Check sheet for the modelled part. Datum: model origin and axes. Units: mm. Face numbers are marked on the shaded views. A direction names the side the tool comes from. Round coordinates to 2 decimals unless told otherwise and drop trailing zeros. Order: outer loops, then holes, each group sorted by start corner. A loop starts at its lowest first (then second) coordinate and runs counter-clockwise, first axis right, second up. Notation, with made-up numbers: M 26,17 L 48,17 A28 ccw 48,47 Z; hole C 7,65.25 d2. An arc over 180 degrees is marked long. One line per item, written item: value. Start each with the question number.
(1) Cross-section at B-B, the plane y = -8. Enter the section's corners in (x, z), and give its area (3 significant figures).
(2) Depth check by flat-ended pin: pin 1 Ø1.5 at (x, y) = (8, -26) entering from +Z; pin 2 Ø1.5 at (x, z) = (3.5, 2) entering from +Y; pin 3 Ø0.9 at (y, z) = (1.5, 1.5) entering from +X; pin 4 Ø0.9 at (x, z) = (1.5, 1.5) entering from -Y. Enter the tip coordinate at first touch or a pass-through.
(3) Release check for a two-part mould opening along X. For the marked faces 1, 2 and 3 record: released by +X, released by -X, zero draft, split by the parting line, or undercut.
(4) Cross-section at A-A, the plane x = 10.2. Enter the section's corners in (y, z), and give its area (3 significant figures).
(5) Cross-section at C-C, the plane z = 2.2. Enter the section's corners in (x, y).
(6) Cross-section at D-D, the plane y = -26. Enter the section's corners in (x, z), and give its area (3 significant figures).
(7) Thickness scan on L1, parallel to Y at x = 10.2, z = 1.95; L2, parallel to X at y = -7.5, z = 1.5; L3, parallel to X at y = 1.5, z = 2.7. Record the ranges inside material, lowest first.
(8) Access from +Z, -Z, +X, -X, +Y, -Y to the whole of each face (thin tool, end or side, straight path). Record for the marked faces 4, 5, 6, 7 and 8.
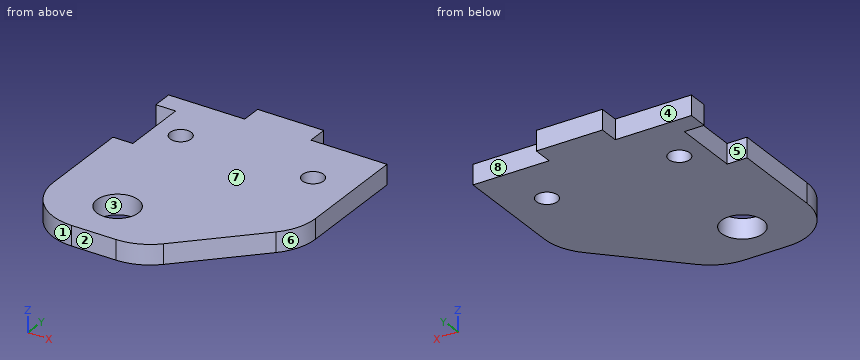
from build123d import *

# Parameters (mm, degrees)
ESBO_O1_R                = 1.6
ESBO_O1_R_2              = 3.15
RESSALTO_EXTRUS_O1_DEPTH = 3
CHANFRO2_SIZE            = 15
FILETE2_R                = 8


with BuildPart() as part:
    # Esboço1 → Ressalto-extrusão1 (new body)
    with BuildSketch(Plane.XY):
        Polygon((11.5, 0), (0, 0), (0, -3), (3, -3), (3, -13), (0, -13), (0, -35), (33, -35), (33, 0), (21.5, 0), (21.5, 3), (11.5, 3), align=None)
        with Locations((27, -8)):
            Circle(ESBO_O1_R, mode=Mode.SUBTRACT)
        with Locations((7, -8)):
            Circle(ESBO_O1_R, mode=Mode.SUBTRACT)
        with Locations((10.2, -27.684295139)):
            Circle(ESBO_O1_R_2, mode=Mode.SUBTRACT)
    extrude(amount=RESSALTO_EXTRUS_O1_DEPTH)

    # Chanfro2
    chanfro2_edges = [part.edges().sort_by_distance(p)[0] for p in [
        (33, -35, 1.5),
    ]]
    chamfer(chanfro2_edges, length=CHANFRO2_SIZE)

    # Filete2
    filete2_edges = [part.edges().sort_by_distance(p)[0] for p in [
        (0, -35, 1.5),
        (33, -20, 1.5),
        (18, -35, 1.5),
    ]]
    fillet(filete2_edges, radius=FILETE2_R)


solid = part.part
Values found:
1. outline: M 3,0 L 5.4,0 L 5.4,3 L 3,3 Z; M 8.6,0 L 25.4,0 L 25.4,3 L 8.6,3 Z; M 28.6,0 L 33,0 L 33,3 L 28.6,3 Z
1. area: 70.8 mm^2
2. pin 1: z = 3
2. pin 2: y = 0
2. pin 3: x = 21.5
2. pin 4: y = -32.23
3. face 1: released by -X
3. face 2: zero draft
3. face 3: undercut
4. outline: M -35,0 L -30.83,0 L -30.83,3 L -35,3 Z; M -24.53,0 L 0,0 L 0,3 L -24.53,3 Z
4. area: 86.1 mm^2
5. outline: M 0,-27 A8 ccw 8,-35 L 14.69,-35 A8 ccw 20.34,-32.66 L 30.66,-22.34 A8 ccw 33,-16.69 L 33,0 L 21.5,0 L 21.5,3 L 11.5,3 L 11.5,0 L 0,0 L 0,-3 L 3,-3 L 3,-13 L 0,-13 Z; hole C 7,-8 d3.2; hole C 10.2,-27.68 d6.3; hole C 27,-8 d3.2
6. outline: M 0,0 L 7.54,0 L 7.54,3 L 0,3 Z; M 12.86,0 L 27,0 L 27,3 L 12.86,3 Z
6. area: 65.0 mm^2
7. L1: -35 to -30.83, -24.53 to 0
7. L2: 3 to 5.48, 8.52 to 25.48, 28.52 to 33
7. L3: 11.5 to 21.5
8. face 4: +Z, -Z, -X, +Y
8. face 5: +Z, -Z, -X
8. face 6: +Z, -Z, +X, -Y
8. face 7: +Z, +X, -X, +Y, -Y
8. face 8: +Z, -Z, +X, +Y
